Here's how the part is built. I have some questions about the finished solid (model axes, mm). Give positions to 0.01 mm unless a question says otherwise; leave off trailing zeros. Loops run counter-clockwise (first coordinate to the right, second up) from the corner with the lowest first, then second, coordinate; pieces in that order, holes last. Notation, with made-up numbers: M 41.25,13.25 L 99.25,13.25 A19 cw 99.25,25.25 Z; hole C 83,69.25 d9. An arc over 180 degrees is marked long. Answer as CSV lines item,"result". Start each with the question number.
Item 1: If I drill on line 1 along Y through (x, z) = (1.5, 9); line 2 along Y through (x, z) = (2, 1.5); line 3 along X through (y, z) = (-6, 13.5), over which ranges is the centre line in solid material (lowest first)? Write a range as from..to.
Item 2: I want a section at B-B on x = 7.5. List the corners of the cut face in (y, z) for me (3 decimals).
Item 3: Will these pins go through, and if not, where does the flat tip stop? P1, Ø8, axis at x = 8, z = 7.5, coming from the +Y side; P2, Ø6, axis at y = -5, z = 4.5, coming from the +X side; P3, Ø3.5, axis at x = 1.15, y = 31.75, coming from the +Z side; P4, Ø1, axis at x = 2.5, z = 8, coming from the -Y side.
Item 4: I want a section at C-C on x = 2.25. List the corners of the cut face in (y, z) for me (3 decimals).
Item 5: I want a section at D-D on y = 25. List the corners of the cut face in (x, z) for me (3 decimals).
Item 6: I want a section at A-A on z = 12.5. List the corners of the cut face in (x, y) for me, plus the area to 3 significant figures.
Item 7: If we mould it in two halves opening along X, with no side actions, what happens to faces 1 (the flat face through (9.036, 28.786, 7.2)), 2 (the cylindrical face through (6.503, 21.876, 7.2)), 3 (the cylindrical face through (0.6, -11.4, 7.2))? For each: released by +X, released by -X, zero draft, split by the parting line, or undercut.
Autodesk Inventor part; units mm, degrees
ref_plane "YZ Plane" through (0, 0, 0) normal (1, 0, 0) x (0, 1, 0)
ref_plane "XZ Plane" through (0, 0, 0) normal (0, 1, 0) x (-1, 0, 0)
ref_plane "XY Plane" through (0, 0, 0) normal (0, 0, 1) x (1, 0, 0)
sketch "Sketch1" plane through (0, 0, 0) normal (0, 0, 1) x (1, 0, 0)
  circle A0 centre (1.1498, 31.75) radius 2.1844
  circle A1 centre (1.1498, -6.35) radius 2.1844
  circle A2 centre (8.2369, 20.5469) radius 2.1844
  arc A3 (-3.9302, -6.35) -> (6.0621, -7.6444) centre (1.1498, -6.35) ccw
  arc A4 (5.4429, 34.4658) -> (-3.9302, 31.75) centre (1.1498, 31.75) ccw
  arc A5 (13.1492, 19.2525) -> (12.53, 23.2627) centre (8.2369, 20.5469) ccw
  line L0 (6.0621, -7.6444) -> (13.1492, 19.2525)
  line L1 (12.53, 23.2627) -> (5.4429, 34.4658)
  line L2 (-3.9302, 31.75) -> (-3.9302, -6.35)
  point P0 (0, 0)
  dimension "d0" = 5.08
  dimension "d1" = 5.08
  dimension "d2" = 5.08
extrude "Extrusion1" add sketch "Sketch1" along normal blind 14.605
properties part number "RoundFix" material "Plastic, Opaque Black"
Result:
1,line 1,"-11.42..-8.51, -4.19..29.59, 33.91..36.82"
1,line 2,"-11.36..-8.36, -4.34..29.74, 33.76..36.76"
1,line 3,"-3.93..-1.01, 3.31..6.5"
2,outline,"M -2.187,0 L 18.491,0 L 18.491,14.605 L -2.187,14.605 Z; M 22.603,0 L 31.214,0 L 31.214,14.605 L 22.603,14.605 Z"
3,P1,"y = 35.96"
3,P2,"x = 7.55"
3,P3,"through"
3,P4,"y = -11.36"
4,outline,"M -11.309,0 L -8.237,0 L -8.237,14.605 L -11.309,14.605 Z; M -4.463,0 L 29.863,0 L 29.863,14.605 L -4.463,14.605 Z; M 33.637,0 L 36.709,0 L 36.709,14.605 L 33.637,14.605 Z"
5,outline,"M -3.93,0 L 11.431,0 L 11.431,14.605 L -3.93,14.605 Z"
6,outline,"M -3.93,-6.35 A5.08 ccw 6.06,-7.64 L 13.15,19.25 A5.08 ccw 12.53,23.26 L 5.44,34.47 A5.08 ccw -3.93,31.75 Z; hole C 1.15,-6.35 d4.37; hole C 1.15,31.75 d4.37; hole C 8.24,20.55 d4.37"
6,area,"573 mm^2"
7,face 1,"released by +X"
7,face 2,"undercut"
7,face 3,"split by the parting line"
